from build123d import *

# Parameters (mm, degrees)
F1_DEPTH = 8.89
F2_DEPTH = 5.08
F3_DEPTH = 2.54


with BuildPart() as f1:
    # F0 (on Top) → F1 (new body)
    with BuildSketch(Plane.XY):
        with BuildLine():
            Line((21.332066, 26.463705), (-27.061316, 57.515545))
            Line((-27.061316, 57.515545), (-28.724159, 0.040585))
            ThreePointArc((-28.724159, 0.040585), (-14.685947, -27.662523), (16.197077, -30.944668))
            Line((16.197077, -30.944668), (43.515381, -48.467725))
            Line((43.515381, -48.467725), (51.195109, -36.495092))
            Line((51.195109, -36.495092), (28.540187, -21.963315))
            ThreePointArc((28.540187, -21.963315), (34.288342, -12.121049), (36.286243, -0.899646))
            ThreePointArc((36.286243, -0.899646), (32.30379, 14.691861), (21.332066, 26.463705))
        make_face()
        with BuildLine():
            Line((-27.236827, 25.100127), (-26.338607, 56.146439))
            Line((-26.338607, 56.146439), (1.208299, 38.470838))
            Line((1.208299, 38.470838), (20.920554, 25.822377))
            ThreePointArc((20.920554, 25.822377), (25.459016, 22.291583), (29.286224, 18.000124))
            ThreePointArc((29.286224, 18.000124), (33.924433, 9.051663), (35.524243, -0.899646))
            ThreePointArc((35.524243, -0.899646), (33.419565, -12.267027), (27.384567, -22.127343))
            Line((27.384567, -22.127343), (28.75755, -23.008029))
            Line((28.75755, -23.008029), (50.142303, -36.725069))
            Line((50.142303, -36.725069), (43.285403, -47.41492))
            Line((43.285403, -47.41492), (17.059054, -30.592287))
            Line((17.059054, -30.592287), (16.271061, -30.086836))
            ThreePointArc((16.271061, -30.086836), (-12.750558, -28.010409), (-27.894731, -3.166497))
            ThreePointArc((-27.894731, -3.166497), (-27.968577, -1.574824), (-27.962478, 0.018549))
            Line((-27.962478, 0.018549), (-27.236827, 25.100127))
        make_face(mode=Mode.SUBTRACT)
    extrude(amount=F1_DEPTH)



with BuildPart() as f2:
    # F0 (on Top) → F2 (new body)
    with BuildSketch(Plane.XY):
        Polygon((-13.605105, 28.150606), (-9.713301, 21.672324), (-7.614988, 18.17948), (-6.73406, 16.713091), (-3.785167, 11.804375), (-2.909715, 10.347101), (0.050701, 5.419203), (0.94598, 3.928926), (3.701448, -0.657816), (4.610738, -2.171416), (7.88597, -7.623355), (8.79526, -9.136955), (10.545028, -12.049613), (18.781333, -25.759736), (19.331383, -26.675345), (20.855503, -25.759736), (20.180433, -24.636017), (12.044667, -11.093252), (10.296888, -8.183906), (9.553734, -6.946853), (6.119241, -1.22981), (5.376086, 0.007243), (2.464367, 4.85408), (1.721212, 6.091132), (-1.380529, 11.254279), (-2.123684, 12.491331), (-5.198242, 17.609229), (-5.941397, 18.846282), (-8.196821, 22.600652), (-12.036798, 28.992664), align=None)
        Polygon((-1.081142, 27.047468), (-5.941397, 18.846282), (-5.198242, 17.609229), (-0.046492, 26.302285), align=None)
        Polygon((4.234035, 23.219336), (-2.123684, 12.491331), (-1.380529, 11.254279), (5.268685, 22.474153), align=None)
        Polygon((9.587057, 19.363947), (1.721212, 6.091132), (2.464367, 4.85408), (10.621708, 18.618764), align=None)
        Polygon((5.376086, 0.007243), (6.119241, -1.22981), (15.710174, 14.953916), (14.675524, 15.699099), align=None)
        Polygon((9.553734, -6.946853), (10.296888, -8.183906), (10.629086, -7.623355), (21.526467, 10.764868), (20.491817, 11.510051), align=None)
        Polygon((-6.73406, 16.713091), (-7.614988, 18.17948), (-16.500566, 19.917602), (-16.744372, 18.671223), (-6.954169, 16.756147), align=None)
        Polygon((-2.909715, 10.347101), (-3.785167, 11.804375), (-16.291279, 14.160487), (-16.526407, 12.912442), align=None)
        Polygon((0.94598, 3.928926), (0.050701, 5.419203), (-16.099113, 8.874321), (-16.364806, 7.632425), (0.701064, 3.981324), align=None)
        Polygon((4.342513, -2.109431), (4.610738, -2.171416), (3.701448, -0.657816), (-15.917408, 3.875942), (-16.203358, 2.638553), align=None)
        Polygon((-15.983448, -3.410797), (8.79526, -9.136955), (7.88597, -7.623355), (-15.697497, -2.173408), align=None)
    extrude(amount=F2_DEPTH)


with BuildPart() as f1_1:
    add(f1.part)

    add(f2.part)  # F3 merges F2
    # F0 (on Top) → F3 (join)
    with BuildSketch(Plane.XY):
        with BuildLine():
            Line((20.920554, 25.822377), (1.208299, 38.470838))
            Line((1.208299, 38.470838), (-8.196821, 22.600652))
            Line((-8.196821, 22.600652), (-5.941397, 18.846282))
            Line((-5.941397, 18.846282), (-1.081142, 27.047468))
            Line((-1.081142, 27.047468), (-0.046492, 26.302285))
            Line((-0.046492, 26.302285), (-5.198242, 17.609229))
            Line((-5.198242, 17.609229), (-2.123684, 12.491331))
            Line((-2.123684, 12.491331), (4.234035, 23.219336))
            Line((4.234035, 23.219336), (5.268685, 22.474153))
            Line((5.268685, 22.474153), (-1.380529, 11.254279))
            Line((-1.380529, 11.254279), (1.721212, 6.091132))
            Line((1.721212, 6.091132), (9.587057, 19.363947))
            Line((9.587057, 19.363947), (10.621708, 18.618764))
            Line((10.621708, 18.618764), (2.464367, 4.85408))
            Line((2.464367, 4.85408), (5.376086, 0.007243))
            Line((5.376086, 0.007243), (14.675524, 15.699099))
            Line((14.675524, 15.699099), (15.710174, 14.953916))
            Line((15.710174, 14.953916), (6.119241, -1.22981))
            Line((6.119241, -1.22981), (9.553734, -6.946853))
            Line((9.553734, -6.946853), (20.491817, 11.510051))
            Line((20.491817, 11.510051), (21.526467, 10.764868))
            Line((21.526467, 10.764868), (10.629086, -7.623355))
            Line((10.629086, -7.623355), (10.296888, -8.183906))
            Line((10.296888, -8.183906), (12.044667, -11.093252))
            Line((12.044667, -11.093252), (29.286224, 18.000124))
            ThreePointArc((29.286224, 18.000124), (25.459016, 22.291583), (20.920554, 25.822377))
        make_face()
        with BuildLine():
            Line((-9.713301, 21.672324), (-27.236827, 25.100127))
            Line((-27.236827, 25.100127), (-27.962478, 0.018549))
            ThreePointArc((-27.962478, 0.018549), (-27.968577, -1.574824), (-27.894731, -3.166497))
            Line((-27.894731, -3.166497), (10.545028, -12.049613))
            Line((10.545028, -12.049613), (8.79526, -9.136955))
            Line((8.79526, -9.136955), (-15.983448, -3.410797))
            Line((-15.983448, -3.410797), (-15.697497, -2.173408))
            Line((-15.697497, -2.173408), (7.88597, -7.623355))
            Line((7.88597, -7.623355), (4.610738, -2.171416))
            Line((4.610738, -2.171416), (4.342513, -2.109431))
            Line((4.342513, -2.109431), (-16.203358, 2.638553))
            Line((-16.203358, 2.638553), (-15.917408, 3.875942))
            Line((-15.917408, 3.875942), (3.701448, -0.657816))
            Line((3.701448, -0.657816), (0.94598, 3.928926))
            Line((0.94598, 3.928926), (0.701064, 3.981324))
            Line((0.701064, 3.981324), (-16.364806, 7.632425))
            Line((-16.364806, 7.632425), (-16.099113, 8.874321))
            Line((-16.099113, 8.874321), (0.050701, 5.419203))
            Line((0.050701, 5.419203), (-2.909715, 10.347101))
            Line((-2.909715, 10.347101), (-16.526407, 12.912442))
            Line((-16.526407, 12.912442), (-16.291279, 14.160487))
            Line((-16.291279, 14.160487), (-3.785167, 11.804375))
            Line((-3.785167, 11.804375), (-6.73406, 16.713091))
            Line((-6.73406, 16.713091), (-6.954169, 16.756147))
            Line((-6.954169, 16.756147), (-16.744372, 18.671223))
            Line((-16.744372, 18.671223), (-16.500566, 19.917602))
            Line((-16.500566, 19.917602), (-7.614988, 18.17948))
            Line((-7.614988, 18.17948), (-9.713301, 21.672324))
        make_face()
        Polygon((28.75755, -23.008029), (27.384567, -22.127343), (20.180433, -24.636017), (20.855503, -25.759736), align=None)
        Polygon((18.781333, -25.759736), (16.271061, -30.086836), (17.059054, -30.592287), (19.331383, -26.675345), align=None)
    extrude(amount=F3_DEPTH)


solid = f1_1.part
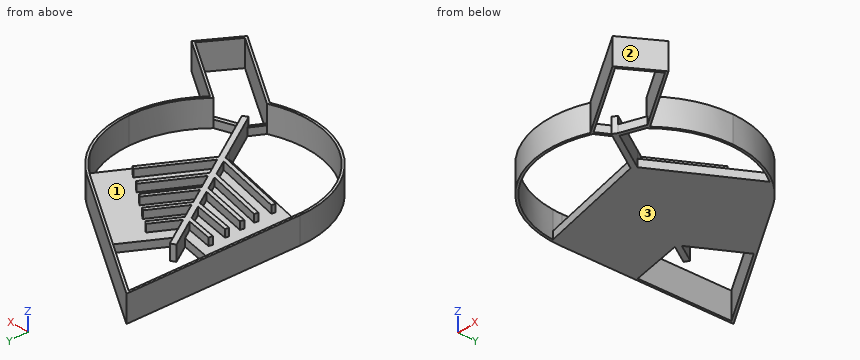
Read the model definition and answer for the solid it produces. Units are mm, in the model's axes. Face numbers are marked on the shaded views. Round coordinates to 2 decimals unless told otherwise and drop trailing zeros. Write each loop counter-clockwise with the first axis right and the second up, starting at its lowest first coordinate (ties: lowest second). Pieces come first, ordered by that corner, then holes.
Q1. Find section B-B on y = 50.5. Determine the outline of the cut face in (x, z).
Values:
outline: (-27.26, 0) - (-26.5, 0) - (-26.5, 8.89) - (-27.26, 8.89) - close; (-17.54, 0) - (-16.13, 0) - (-16.13, 8.89) - (-17.54, 8.89) - close
Q2. Find section C-C on x = 46.5. Determine the outline of the cut face in (y, z).
Values:
outline: (-43.81, 0) - (-42.4, 0) - (-42.4, 8.89) - (-43.81, 8.89) - close; (-34.39, 0) - (-33.48, 0) - (-33.48, 8.89) - (-34.39, 8.89) - close
Q3. Find section A-A on z = 7. Determine the outline of the cut face in (x, y).
Values:
outline: (-28.72, 0.04) arc R32.51 ccw to (16.2, -30.94) - (43.52, -48.47) - (51.2, -36.5) - (28.54, -21.96) arc R32.51 ccw to (36.29, -0.9) arc R32.51 ccw to (21.33, 26.46) - (-27.06, 57.52) - close; hole (-27.96, 0.02) arc R31.75 ccw to (-27.89, -3.17) arc R31.75 ccw to (16.27, -30.09) - (17.06, -30.59) - (43.29, -47.41) - (50.14, -36.73) - (28.76, -23.01) - (27.38, -22.13) arc R31.75 ccw to (35.52, -0.9) arc R31.75 ccw to (29.29, 18) arc R31.75 ccw to (20.92, 25.82) - (-26.34, 56.15) - close
Q4. Straight lines are drawn through the part: line 1 (X direction, y = 9.5, z = 4); line 2 (Y direction, x = 0.5, z = 1.5); line 3 (Y direction, x = 33, z = 7.5). For each, find the intervals that lie inside material, in ascending order.
Values:
line 1: x = -28.45 to -27.69, -2.4 to -0.33, 3.74 to 5.22, 11 to 12.48, 19.3 to 20.78, 33.77 to 34.58
line 2: y = -33.25 to -32.48, -9.73 to 37.28, 38.93 to 39.83
line 3: y = -41.72 to -40.82, -25.73 to -24.82, -15.14 to -13.31, 11.51 to 13.34
Q5. Flat-ended cylindrical pins translate along their axes: P1, Ø5, axis at x = 37, z = 5.5, coming from the -Y side; P2, Ø4, axis at x = 24.5, z = 2.5, coming from the +Y side; P3, Ø11, axis at x = 7.5, y = 13.5, coming from the +Z side. Find the tip coordinate at first contact, or state that the pin passes through.
Values:
P1: stops at y = -45.89
P2: stops at y = 25.68
P3: stops at z = 5.08
Q6. The mould has two halves that part along X. Classify the marked faces 1, 2 and 3: released by +X, released by -X, zero draft, split by the parting line, or undercut.
Values:
face 1: undercut
face 2: released by +X
face 3: zero draft
